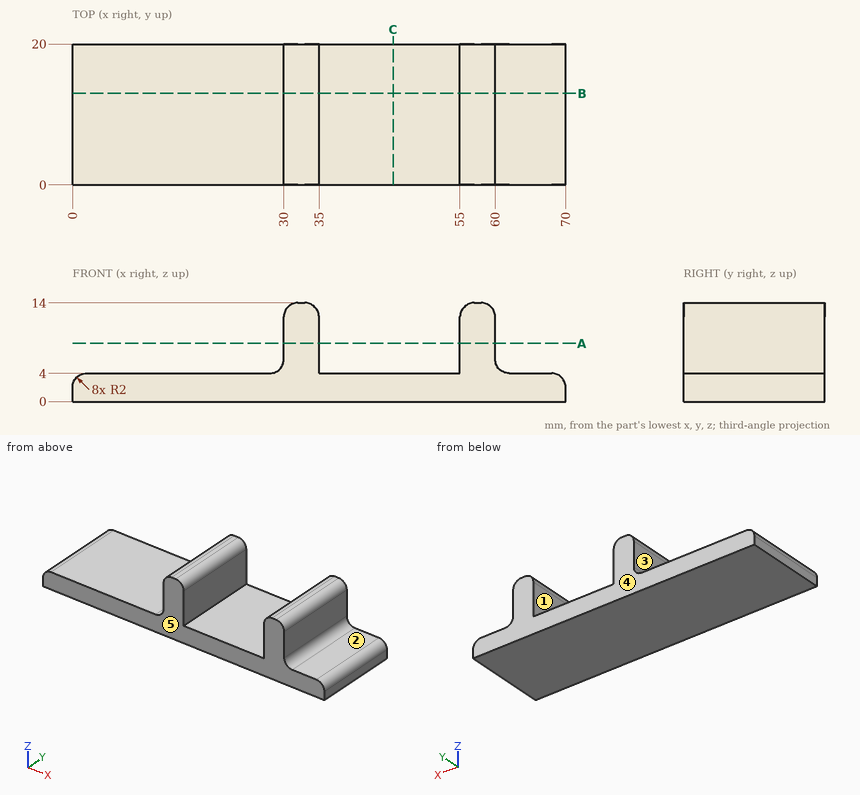
Study the drawing (mm; zero at the part's minimum x, y, z) and answer. A direction names the side the tool comes from. Round coordinates to 2 decimals unless told otherwise and drop trailing zeros. Write each loop counter-clockwise with the first axis right and the second up, starting at its lowest first coordinate (ties: lowest second). Pieces come first, ordered by that corner, then holes. Notation, with made-up numbers: (-12, 59) - (29, 59) arc R30 ccw to (29, 88) - close; hole circle Ø7 at (73, 23.25). An arc over 180 degrees is marked (long way). Return JSON: item names as keys, results as strings. Group by question number.
Q1. The part is cut by section C-C on x = 45.5. Write down the section's boundary in (y, z), then the cut area to 3 significant figures.
Q2. The part is cut by section A-A on z = 8.25. Write down the section's boundary in (x, y), then the cut area to 3 significant figures.
Q3. Each of these flat-tipped pins is pushed along its axis until it touches: pin 1 Ø10 at (x, y) = (14.5, 14) entering from +Z; pin 2 Ø1.5 at (x, y) = (55, 15.5) entering from +Z; pin 3 Ø4 at (y, z) = (6, 11) entering from +X. Where does it stop, or does it pass through?
Q4. The part is cut by section B-B on y = 13. Write down the section's boundary in (x, z), then the cut area to 3 significant figures.
Q5. For the marked faces 1, 2, 3, 4 and 5, determine the directions among +Z, -Z, +X, -X, +Y, -Y from which every point of the face is accessible in a straight line to the end or side of a thin tool.
Q6. Find the intervals of material crossed by L1, parallel to X at y = 11.25, z = 7.75; L2, parallel to Z at x = 46, y = 4.5; L3, parallel to X at y = 13.75, z = 4.5, in increasing order.
Solved:
{
 "1": {"outline": "(0, 0) - (20, 0) - (20, 4) - (0, 4) - close", "area": "80.0 mm²"},
 "2": {"outline": "(30, 0) - (35, 0) - (35, 20) - (30, 20) - close; (55, 0) - (60, 0) - (60, 20) - (55, 20) - close", "area": "200 mm²"},
 "3": {"pin 1": "z = 4", "pin 2": "z = 13.56", "pin 3": "x = 60"},
 "4": {"outline": "(0, 0) - (70, 0) - (70, 2) arc R2 ccw to (68, 4) - (62, 4) arc R2 cw to (60, 6) - (60, 12) arc R2 ccw to (58, 14) - (57, 14) arc R2 ccw to (55, 12) - (55, 4) - (35, 4) - (35, 12) arc R2 ccw to (33, 14) - (32, 14) arc R2 ccw to (30, 12) - (30, 6) arc R2 cw to (28, 4) - (2, 4) arc R2 ccw to (0, 2) - close", "area": "377 mm²"},
 "5": {"face 1": "+Z, +Y, -Y", "face 2": "+Z, +X, +Y, -Y", "face 3": "+Z, -X, +Y, -Y", "face 4": "+Z, -Z, +X, -X, +Y", "face 5": "+Z, -Z, +X, -X, -Y"},
 "6": {"L1": "30 to 35, 55 to 60", "L2": "0 to 4", "L3": "29.32 to 35, 55 to 60.68"}
}
